Autodesk Inventor part; units mm, degrees
ref_plane "YZ Plane" through (0, 0, 0) normal (1, 0, 0) x (0, 1, 0)
ref_plane "XZ Plane" through (0, 0, 0) normal (0, 1, 0) x (-1, 0, 0)
ref_plane "XY Plane" through (0, 0, 0) normal (0, 0, 1) x (1, 0, 0)
sketch "Sketch1" plane through (0, 0, 0) normal (0, 0, 1) x (1, 0, 0)
  arc A0 (-5.5, 2.3979) -> (5.5, 2.3979) centre (0, 0) ccw
  line L0 (-8.5, 0) -> (-8.5, 25)
  line L1 (-8.5, 25) -> (-5.5, 25)
  line L2 (-5.5, 25) -> (-5.5, 2.3979)
  line L3 (5.5, 2.3979) -> (5.5, 25)
  line L4 (5.5, 25) -> (8.5, 25)
  line L5 (8.5, 25) -> (8.5, 0)
  arc A1 (-8.5, 0) -> (8.5, 0) centre (0, 0) ccw
  dimension "d0" = 12
  dimension "d2" = 25
  dimension "d4" = 3
  dimension "d5" = 3
  dimension "d6" = 8.5
extrude "Extrusion1" add sketch "Sketch1" along normal blind 16
fillet "Fillet1" radius 6 4 edges at (-7, 25, 16) (-7, 25, 0) (7, 25, 0) (7, 25, 16)
sketch "Sketch2" plane through (-8.5, 0, 0) normal (-1, 0, 0) x (0, 0, 1)
  circle A0 centre (5, -2.5) radius 1.4
  circle A1 centre (5, 7.025) radius 1.4
  line L0 (0, 0) -> (0, 19)
  line L1 (0, -8.5) -> (16, -8.5)
  dimension "d10" = 2.8
  dimension "d11" = 2.8
  dimension "d12" = 9.525
  dimension "d13" = 5
  dimension "d14" = 6
extrude "Extrusion2" add sketch "Sketch2" along normal blind 7
sketch "Sketch3" plane through (0, 0, 0) normal (0, 0, -1) x (-1, 0, 0)
  line L0 (-8.5, 19) -> (-5.5, 19)
  line L1 (-8.5, 19) -> (-8.5, 0)
  arc A0 (-8.5, 0) -> (8.5, 0) centre (0, 0) ccw
  line L2 (8.5, 0) -> (8.5, 19)
  line L3 (5.5, 19) -> (8.5, 19)
  line L4 (5.5, 19) -> (5.5, 2.3979)
  arc A1 (-5.5, 2.3979) -> (5.5, 2.3979) centre (0, 0) ccw
  line L5 (-5.5, 2.3979) -> (-5.5, 19)
  line L6 (8.5, 0) -> (8.5, -8.5)
  arc A2 (-8.5, 0) -> (8.5, 0) centre (0, 0) ccw
  line L7 (8.5, -1.1) -> (8.5, -3.9)
  line L8 (8.5, -8.5) -> (-8.5, -8.5)
  line L9 (-8.5, 0) -> (-8.5, -8.5)
  line L10 (8.5, 0) -> (6, 0)
  line L11 (-8.5, 19) -> (-8.5, 0)
  line L12 (-6, 0) -> (-8.5, 0)
extrude "Extrusion3" add sketch "Sketch3" against normal up to surface (16 mm away) contours A0 L8 L9 | A0 L6 L8
fillet "Fillet2" radius 4 2 edges at (-8.5, -8.5, 8) (8.5, -8.5, 8)
hole "Hole1" at (-8.5, 19, 8) direction (1, 0, 0) diameter 3 end through all
sketch "Sketch5" plane through (8.5, 25, 10) normal (1, 0, 0) x (0, 0, -1)
  circle A0 centre (2, -6) radius 1.5
  line L0 (10, -29.5) -> (-6, -29.5)
  line L1 (10, -6) -> (10, -29.5)
  arc A1 (10, -6) -> (4, 0) centre (4, -6) ccw
  line L2 (4, 0) -> (0, 0)
  arc A2 (0, 0) -> (-6, -6) centre (0, -6) ccw
  line L3 (-6, -6) -> (-6, -29.5)
  line L4 (5.2332, -6) -> (3.6166, -8.8)
  line L5 (3.6166, -8.8) -> (0.3834, -8.8)
  line L6 (0.3834, -8.8) -> (-1.2332, -6)
  line L7 (-1.2332, -6) -> (0.3834, -3.2)
  line L8 (0.3834, -3.2) -> (3.6166, -3.2)
  line L9 (3.6166, -3.2) -> (5.2332, -6)
  point P0 (10, -25)
  dimension "d29" = 5.6
extrude "Extrusion4" cut sketch "Sketch5" against normal blind 1 contours L4 L5 L6 L7 L8 L9
sketch "Sketch6" plane through (0, 0, 0) normal (0, 0, -1) x (-1, 0, 0)
  arc A0 (-8.5, -4.5) -> (-4.5, -8.5) centre (-4.5, -4.5) ccw
  line L0 (-4.5, -8.5) -> (4.5, -8.5)
  arc A1 (4.5, -8.5) -> (8.5, -4.5) centre (4.5, -4.5) ccw
  line L1 (8.5, -4.5) -> (8.5, 19)
  line L2 (5.5, 19) -> (8.5, 19)
  line L3 (5.5, 19) -> (5.5, 2.3979)
  arc A2 (-5.5, 2.3979) -> (5.5, 2.3979) centre (0, 0) ccw
  line L4 (-5.5, 2.3979) -> (-5.5, 19)
  line L5 (-8.5, 19) -> (-5.5, 19)
  line L6 (-8.5, 19) -> (-8.5, -4.5)
  line L7 (15.5, 5.625) -> (15.5, 8.425)
  line L8 (8.5, 8.425) -> (8.5, 5.625)
  line L9 (15.5, -3.9) -> (15.5, -1.1)
  line L10 (8.5, -1.1) -> (8.5, -3.9)
  line L11 (8.5, 8.425) -> (15.5, 8.425)
  line L12 (8.5, 5.625) -> (15.5, 5.625)
  line L13 (8.5, -1.1) -> (15.5, -1.1)
  line L14 (8.5, -3.9) -> (15.5, -3.9)
  line L15 (8.5, 10) -> (15.5, 10)
  line L16 (15.5, 10) -> (15.5, 4)
  line L17 (15.5, 4) -> (8.5, 4)
  line L18 (8.5, 4) -> (8.5, 10)
  line L19 (8.5, 19) -> (8.5, -4.5)
  line L20 (8.5, 1) -> (15.5, 1)
  line L21 (15.5, 1) -> (15.5, -6.597)
  line L22 (15.5, -6.597) -> (8.5, -6.597)
  line L23 (8.5, -6.597) -> (8.5, 1)
extrude "Extrusion6" add sketch "Sketch6" against normal blind 3.5 contours L1 L14 L21 L22 L23 | L1 L20 L21 L13 | L1 L12 L16 L17 | L15 L16 L11 L1
sketch "Sketch7" plane through (0, 0, 3.5) normal (0, 0, 1) x (1, 0, 0)
  line L0 (-8.5, 5.625) -> (-15.5, 5.625)
  line L1 (-15.5, 5.625) -> (-15.5, 4)
  line L2 (-15.5, 4) -> (-8.5, 4)
  line L3 (-8.5, 5.625) -> (-8.5, 4)
  line L4 (-15.5, 8.425) -> (-8.5, 8.425)
  line L5 (-8.5, 10) -> (-8.5, 5.625)
  line L6 (-8.5, 10) -> (-15.5, 10)
  line L7 (-15.5, 10) -> (-15.5, 5.625)
  line L8 (-15.5, -1.1) -> (-8.5, -1.1)
  line L9 (-8.5, 1) -> (-8.5, -3.9)
  line L10 (-8.5, 1) -> (-15.5, 1)
  line L11 (-15.5, 1) -> (-15.5, -3.9)
  line L12 (-8.5, -3.9) -> (-15.5, -3.9)
  line L13 (-15.5, -3.9) -> (-15.5, -6.597)
  line L14 (-15.5, -6.597) -> (-8.5, -6.597)
  line L15 (-8.5, -6.597) -> (-8.5, -4.5)
  line L16 (-8.5, -3.9) -> (-8.5, -4.5)
  line L17 (-8.5, 8.425) -> (-7, 6)
  line L18 (-8.5, 5.625) -> (-15.5, 5.625)
  point P0 (0, 0)
extrude "Extrusion7" add sketch "Sketch7" against normal blind 0.5 contours L0 L7 L4 L5 | L8 L9 L12 L11
properties part number "microswitch 12mm axe support"
Read the model definition and answer for the solid it produces. Units are mm, in the model's axes. A direction names the side the tool comes from. Coordinates: 2 decimals unless noted, no trailing zeros. Write each loop counter-clockwise with the first axis right and the second up, starting at its lowest first coordinate (ties: lowest second). Pieces come first, ordered by that corner, then holes. Notation, with made-up numbers: (35.25, -40) - (92.25, -40) arc R13 cw to (92.25, -17) - close; hole circle Ø5 at (-36, 68). An arc over 180 degrees is marked (long way). Answer as a JSON object with one key per item and string values. Group by question number.
1. A cutting plane is placed at A-A (y = 0). Determine the outline of the cut face in (x, z).
2. A cutting plane is placed at C-C (y = 3.5). Determine the outline of the cut face in (x, z).
3. A cutting plane is placed at D-D (x = 0). Determine the outline of the cut face in (y, z), plus the area to 3 significant figures.
4. A cutting plane is placed at B-B (z = 8). Determine the outline of the cut face in (x, y).
5. The mould has two halves that part along Y. Classify faces 1 (the cylindrical face through (-11.951, 7.561, 6.293)), 2 (the flat face through (-6, 2, 0)), 3 (the cylindrical face through (7.021, 23.289, 14.196)): +Y half, -Y half, draft (parallel to the pull), parting line (faces both ways), or undercut.
6. Consider L1, parallel to Y at x = -14.25, z = 1.5 (3 decimals); L2, parallel to X at y = 17, z = 11.75; L3, parallel to X at y = 0, z = 9. Determine where each line is inside the solid, lowest interval first. Write a range as [from, to].
7. Each of these flat-tipped pins is pushed along its axis until it touches: P1, Ø2, axis at y = -3, z = 1, coming from the -X side; P2, Ø5, axis at y = 13.5, z = 11.5, coming from the -X side; P3, Ø2, axis at x = -12.5, y = -1.5, coming from the +Z side; P4, Ø0.9, axis at x = -10.5, z = 2, coming from the -Y side. Where does it stop, or does it pass through?
8. Which of the six approach directions +Z, -Z, +X, -X, +Y, -Y give full straight-line access (tool end or side, diameter ignored) to faces 4 (the flat face through (-12, 6, 3.5)), 5 (the flat face through (-12, 4, 2)), 6 (the flat face through (8, 16.2, 8))?
Worked out:
{
 "1": {"outline": "(-15.5, 0) - (-6, 0) - (-6, 16) - (-8.5, 16) - (-8.5, 3.5) - (-15.5, 3.5) - close; (6, 0) - (8.5, 0) - (8.5, 16) - (6, 16) - close"},
 "2": {"outline": "(-8.5, 0) - (-5.5, 0) - (-5.5, 16) - (-8.5, 16) - close; (5.5, 0) - (8.5, 0) - (8.5, 16) - (5.5, 16) - close"},
 "3": {"outline": "(-8.5, 0) - (-6, 0) - (-6, 16) - (-8.5, 16) - close", "area": "40.0 mm²"},
 "4": {"outline": "(-8.5, -4.5) arc R4 ccw to (-4.5, -8.5) - (4.5, -8.5) arc R4 ccw to (8.5, -4.5) - (8.5, 16.2) - (7.5, 16.2) - (7.5, 17.5) - (5.5, 17.5) - (5.5, 2.4) arc R6 cw (long way) to (-5.5, 2.4) - (-5.5, 17.5) - (-8.5, 17.5) - close; (-8.5, 20.5) - (-5.5, 20.5) - (-5.5, 25) - (-8.5, 25) - close; (5.5, 20.5) - (7.5, 20.5) - (7.5, 21.8) - (8.5, 21.8) - (8.5, 25) - (5.5, 25) - close"},
 "5": {"face 1": "undercut", "face 2": "draft", "face 3": "+Y half"},
 "6": {"L1": "y = [-6.597, -3.9], [-1.1, 1], [4, 5.625], [8.425, 10]", "L2": "x = [-8.5, -5.5], [5.5, 8.5]", "L3": "x = [-8.5, -6], [6, 8.5]"},
 "7": {"P1": "stops at x = -15.5", "P2": "stops at x = -8.5", "P3": "stops at z = 6.4", "P4": "stops at y = -6.6"},
 "8": {"face 4": "-X, +Y, -Y", "face 5": "+Z, -Z, -X", "face 6": "+X"}
}
